from build123d import *

# Parameters (mm, degrees)
BOSS_EXTRUDE1_DEPTH = 152.4
BOSS_EXTRUDE2_DEPTH = 12.7
BOSS_EXTRUDE4_DEPTH = 12.7


with BuildPart() as part:
    # Sketch1 → Boss-Extrude1 (new body)
    with BuildSketch(Plane.XY):
        Polygon((-67.57780806, 32.405365497), (237.22219194, 32.405365497), (203.770487766, -29.214920061), (-50.229512234, -29.214920061), align=None)
    extrude(amount=BOSS_EXTRUDE1_DEPTH)

    # Sketch2 → Boss-Extrude2 (add)
    with BuildSketch(Plane.XY.offset(152.4)):
        Polygon((181.065122105, -29.214920061), (214.407517956, 32.405365497), (207.478022529, 32.405365497), (174.135626677, -29.214920061), align=None)
        Polygon((166.529193842, -29.214920061), (199.871589694, 32.405365497), (192.204880741, 32.405365497), (158.862484889, -29.214920061), align=None)
        Polygon((151.231941607, -29.214920061), (184.574337458, 32.405365497), (176.954337458, 32.405365497), (143.611941607, -29.214920061), align=None)
    extrude(amount=BOSS_EXTRUDE2_DEPTH)

    # Sketch4 → Boss-Extrude4 (add)
    with BuildSketch(Plane(origin=(0, 0, 0), x_dir=(-1, 0, 0), z_dir=(0, 0, -1))):
        Polygon((-181.966188402, 32.405365497), (-151.231941607, -29.214920061), (-143.611941607, -29.214920061), (-174.485930726, 32.405365497), align=None)
        Polygon((-197.403182961, 32.405365497), (-166.529193842, -29.214920061), (-158.862484889, -29.214920061), (-190.426148903, 32.405365497), align=None)
        Polygon((-213.709292703, 32.405365497), (-181.065122105, -29.214920061), (-174.135626677, -29.214920061), (-205.699290692, 32.405365497), align=None)
    extrude(amount=BOSS_EXTRUDE4_DEPTH)


solid = part.part
The listing builds one solid part. Answer for the finished solid, in the listing's coordinates (mm). A direction names the side the tool comes from. Coordinates: 2 decimals unless noted, no trailing zeros. Loops run counter-clockwise (first coordinate to the right, second up) from the corner with the lowest first, then second, coordinate; pieces in that order, holes last. Notation, with made-up numbers: (-37, 23.25) -> (-16, 23.25) arc R22 cw to (-16, 43.25) -> close; hole circle Ø6 at (19, -11). An arc over 180 degrees is marked (long way). Answer in a Markdown table with one row per item. Add a question column.
1. The part is cut by section C-C, the plane z = 118. Write down the section's boundary in (x, y), then the cut area to 3 significant figures.
2. Determine the mould class of faces 5 (the flat face through (191.04, 2.03, 158.66)), 6 (the flat face through (220.731, 2.027, 75.133)), 7 (the flat face through (177, 2, -12.7)) for opening direction Y: +Y half, -Y half, draft (parallel to the pull), parting line (faces both ways), or undercut.
3. For faces 1 (the flat face through (182.967, 1.164, 158.661)), 2 (the flat face through (197.5, 1.16, 158.66)), 3 (the flat face through (158.83, 1.16, -6.26)), 4 (the flat face through (189.697, 1.164, -6.261)), determine the directions among +Z, -Z, +X, -X, +Y, -Y from which every point of the face is accessible in a straight line to the end or side of a thin tool.
4. Consider line 1 (X direction, y = -24, z = -5); line 2 (Z direction, x = 16.5, y = -1.5); line 3 (X direction, y = -10, z = 154). Determine where each line is inside the solid, lowest interval first. Write a range as [from, to].
5. The part is cut by section B-B, the plane x = 46.5. Write down the section's boundary in (y, z), then the cut area to 3 significant figures.
6. The part is cut by section A-A, the plane y = 25. Write down the section's boundary in (x, z).
7. The part is cut by section D-D, the plane y = -8. Write down the section's boundary in (x, z).
8. Flat-ended cylindrical pins translate along their axes: P1, Ø17, axis at x = 214, y = 2, coming from the -Z side; P2, Ø1.5, axis at x = 137, y = 24.5, coming from the +Z side; P3, Ø3, axis at y = -12.5, z = 83.5, coming from the +X side. Find the tip coordinate at first contact, or state that the pin passes through.
Answer below:
| question | item | result |
|---|---|---|
| 1 | outline | (-67.58, 32.41) -> (-50.23, -29.21) -> (203.77, -29.21) -> (237.22, 32.41) -> close |
| 1 | area | 17,200 mm2 |
| 2 | face 5 | undercut |
| 2 | face 6 | -Y half |
| 2 | face 7 | draft |
| 3 | face 1 | +Z |
| 3 | face 2 | +Z, +X, -Y |
| 3 | face 3 | -Z, -X, +Y |
| 3 | face 4 | -Z |
| 4 | line 1 | [146.22, 153.83], [161.53, 169.14], [176.81, 183.83] |
| 4 | line 2 | [0, 152.4] |
| 4 | line 3 | [154.01, 161.63], [169.26, 176.93], [184.53, 191.46] |
| 5 | outline | (-29.21, 0) -> (32.41, 0) -> (32.41, 152.4) -> (-29.21, 152.4) -> close |
| 5 | area | 9,390 mm2 |
| 6 | outline | (-65.49, 0) -> (170.78, 0) -> (170.78, -12.7) -> (178.27, -12.7) -> (178.27, 0) -> (186.63, 0) -> (186.63, -12.7) -> (193.69, -12.7) -> (193.69, 0) -> (201.91, 0) -> (201.91, -12.7) -> (209.79, -12.7) -> (209.79, 0) -> (233.2, 0) -> (233.2, 152.4) -> (210.4, 152.4) -> (210.4, 165.1) -> (203.47, 165.1) -> (203.47, 152.4) -> (195.86, 152.4) -> (195.86, 165.1) -> (188.2, 165.1) -> (188.2, 152.4) -> (180.57, 152.4) -> (180.57, 165.1) -> (172.95, 165.1) -> (172.95, 152.4) -> (-65.49, 152.4) -> close |
| 7 | outline | (-56.2, 0) -> (154.24, 0) -> (154.24, -12.7) -> (161.81, -12.7) -> (161.81, 0) -> (169.73, 0) -> (169.73, -12.7) -> (177.16, -12.7) -> (177.16, 0) -> (185, 0) -> (185, -12.7) -> (192.3, -12.7) -> (192.3, 0) -> (215.29, 0) -> (215.29, 152.4) -> (192.54, 152.4) -> (192.54, 165.1) -> (185.61, 165.1) -> (185.61, 152.4) -> (178.01, 152.4) -> (178.01, 165.1) -> (170.34, 165.1) -> (170.34, 152.4) -> (162.71, 152.4) -> (162.71, 165.1) -> (155.09, 165.1) -> (155.09, 152.4) -> (-56.2, 152.4) -> close |
| 8 | P1 | z = 0 |
| 8 | P2 | z = 152.4 |
| 8 | P3 | x = 213.66 |
